from build123d import *

# Parameters (mm, degrees)
F1_DEPTH = 3.5
F2_R     = 1.5
F3_DEPTH = 2


# Not quite as in the source:
# - a feature names something its author has since deleted; it is built from what else it names


with BuildPart() as f1:
    # F0 (on Front) → F1 (new body)
    with BuildSketch(Plane.XZ):
        Polygon((42.7356177972, 8.1960540903), (-9.8386000647, 97.8239037067), (-62.5526416078, 8.1960540903), align=None)
        with BuildLine():
            Line((-12.7572676559, 11.6960540903), (-56.4336672666, 11.6960540903))
            Line((-56.4336672666, 11.6960540903), (-35.4842691453, 47.3155863706))
            ThreePointArc((-35.4842691453, 47.3155863706), (-32.6024132797, 24.0941164977), (-12.7572676559, 11.6960540903))
        make_face(mode=Mode.SUBTRACT)
        with BuildLine():
            ThreePointArc((-11.7914030425, 15.1152742164), (-33.3740588193, 38.7305133045), (-11.7914030425, 62.3457523925))
            Line((-11.7914030425, 62.3457523925), (-11.7914030425, 15.1152742164))
        make_face(mode=Mode.SUBTRACT)
        with BuildLine():
            ThreePointArc((-6.5689498166, 11.6960540903), (13.2761958072, 24.0941164977), (16.1580516728, 47.3155863706))
            Line((16.1580516728, 47.3155863706), (37.1074497941, 11.6960540903))
            Line((37.1074497941, 11.6960540903), (-6.5689498166, 11.6960540903))
        make_face(mode=Mode.SUBTRACT)
        with BuildLine():
            ThreePointArc((-7.8989818992, 62.3757456007), (14.0478413468, 38.7305133045), (-7.8989818992, 15.0852810082))
            Line((-7.8989818992, 15.0852810082), (-7.8989818992, 62.3757456007))
        make_face(mode=Mode.SUBTRACT)
        with BuildLine():
            Line((-29.7147789735, 57.1252496473), (-11.7914030425, 87.5997417472))
            Line((-11.7914030425, 87.5997417472), (-11.7914030425, 65.8581038309))
            ThreePointArc((-11.7914030425, 65.8581038309), (-21.5817241061, 63.1923695727), (-29.7147789735, 57.1252496473))
        make_face(mode=Mode.SUBTRACT)
        with BuildLine():
            Line((-7.8989818992, 65.8842176728), (-7.8989818992, 87.5997417472))
            Line((-7.8989818992, 87.5997417472), (9.3459755849, 58.2007602904))
            ThreePointArc((9.3459755849, 58.2007602904), (1.4112063573, 63.5860026304), (-7.8989818992, 65.8842176728))
        make_face(mode=Mode.SUBTRACT)
    extrude(amount=F1_DEPTH)

    # F2 (on face) → F3 (join)
    with BuildSketch(Plane(origin=(0, 0, 8.1960540903), x_dir=(1, 0, 0), z_dir=(0, 0, -1))):
        with Locations((-9.9085119053, 1.75)):
            Circle(F2_R)
    extrude(amount=F3_DEPTH)


solid = f1.part
Verification items for the finished model (mm, model axes). A direction names the side the tool comes from. Coordinates: 2 decimals unless noted, no trailing zeros. Loops run counter-clockwise (first coordinate to the right, second up) from the corner with the lowest first, then second, coordinate; pieces in that order, holes last. Notation, with made-up numbers: (64, 53) -> (93, 53) arc R24 ccw to (93, 66) -> close; hole circle Ø8 at (76, 52.25). An arc over 180 degrees is marked (long way). Answer as CSV lines item,"result".
1) Cross-section at A-A, the plane y = -1.75. Record the cut outline in (x, z).
Found:
outline,"(-62.55, 8.2) -> (-11.41, 8.2) -> (-11.41, 6.2) -> (-8.41, 6.2) -> (-8.41, 8.2) -> (42.74, 8.2) -> (-9.84, 97.82) -> close; hole (-56.43, 11.7) -> (-12.76, 11.7) arc R27.21 cw to (-35.48, 47.32) -> close; hole (-29.71, 57.13) arc R27.21 cw to (-11.79, 65.86) -> (-11.79, 87.6) -> close; hole (-11.79, 15.12) -> (-11.79, 62.35) arc R23.71 ccw to start; hole (-7.9, 15.09) arc R23.71 ccw to (-7.9, 62.38) -> close; hole (-7.9, 65.88) arc R27.21 cw to (9.35, 58.2) -> (-7.9, 87.6) -> close; hole (-6.57, 11.7) -> (37.11, 11.7) -> (16.16, 47.32) arc R27.21 cw to start"
2) Tool access check on faces 1 (the flat face through (-46.106, -1.726, 29.256)), 2 (the flat face through (-35.827, -1.726, 53.637)). Record the directions out of +Z, -Z, +X, -X, +Y, -Y that give a thin tool (end or side, any length) a straight path to the whole face; none if there is none.
Found:
face 1,"+Y, -Y"
face 2,"+Z, -X, +Y, -Y"
3) Cross-section at D-D, the plane x = -32. Record the cut outline in (y, z), then the cut area to 3 significant figures.
Found:
outline,"(-3.5, 8.2) -> (0, 8.2) -> (0, 11.7) -> (-3.5, 11.7) -> close; (-3.5, 23.19) -> (0, 23.19) -> (0, 30.78) -> (-3.5, 30.78) -> close; (-3.5, 46.68) -> (0, 46.68) -> (0, 60.14) -> (-3.5, 60.14) -> close"
area,"85.9 mm2"
4) Cross-section at B-B, the plane z = 41.5. Record the cut outline in (x, y).
Found:
outline,"(-42.97, -3.5) -> (-38.9, -3.5) -> (-38.9, 0) -> (-42.97, 0) -> close; (-36.73, -3.5) -> (-33.21, -3.5) -> (-33.21, 0) -> (-36.73, 0) -> close; (-11.79, -3.5) -> (-7.9, -3.5) -> (-7.9, 0) -> (-11.79, 0) -> close; (13.89, -3.5) -> (17.41, -3.5) -> (17.41, 0) -> (13.89, 0) -> close; (19.58, -3.5) -> (23.2, -3.5) -> (23.2, 0) -> (19.58, 0) -> close"
5) Thickness scan on L1, parallel to X at y = -1.85, z = 53.5; L2, parallel to X at y = -2.6, z = 69; L3, parallel to Z at x = -27, y = -1.4. Record the ranges inside material, lowest first. Write a range as from..to.
Found:
L1,"x = -35.91..-28.21, -11.79..-7.9, 8.89..16.16"
L2,"x = -26.79..-22.73, -11.79..-7.9, 3.01..7.07"
L3,"z = 8.2..11.7, 17.76..22.56, 54.91..59.7, 61.74..68.64"
6) Depth check by flat-ended pin: pin 1 (1 mm diameter, centred on y = -1, z = 72, fed in from -X); pin 2 (1 mm diameter, centred on y = -2, z = 18, fed in from +X); pin 3 (1.8 mm diameter, centred on y = -2, z = 41.5, fed in from -X); pin 4 (4 mm diameter, centred on x = 2, z = 17, fed in from +Y). Enter the tip coordinate at first touch or a pass-through.
Found:
pin 1,"stops at x = -25.32"
pin 2,"stops at x = 37.28"
pin 3,"stops at x = -43.49"
pin 4,"stops at y = 0"
7) Release check for a two-part mould opening along X. For faces 3 (the flat face through (26.486, -1.726, 29.755)), 4 (the cylindrical face through (-8.478, -2.201, 7.21)), 5 (the flat face through (-10, -2, 6.196)) record: +X half, -X half, draft (parallel to the pull), parting line (faces both ways), or undercut.
Found:
face 3,"undercut"
face 4,"parting line"
face 5,"draft"
8) Cross-section at C-C, the plane x = 33. Record the cut outline in (y, z), then the cut area to 3 significant figures.
Found:
outline,"(-3.5, 8.2) -> (0, 8.2) -> (0, 11.7) -> (-3.5, 11.7) -> close; (-3.5, 18.68) -> (0, 18.68) -> (0, 24.79) -> (-3.5, 24.79) -> close"
area,"33.6 mm2"
